from build123d import *

# Parameters (mm, degrees)
F0_W     = 381
F0_H     = 342.9
F1_DEPTH = 330.2
F2_T     = -6.35
F4_DEPTH = 12.7
F5_R     = 6.35
F6_DEPTH = 3.175
F7_R     = 12.7
F8_DEPTH = 12.7
F9_R     = 5.08


with BuildPart() as f1:
    # F0 (on Top) → F1 (new body)
    with BuildSketch(Plane.XY):
        with Locations((83.37315, 21.438057)):
            Rectangle(F0_W, F0_H)
    extrude(amount=F1_DEPTH)

    # F2
    f2_openings = [f1.faces().sort_by_distance(p)[0] for p in [
        (83.37315, 21.438057, 330.2),
    ]]
    offset(amount=F2_T, openings=f2_openings)

    # F3 (on face) → F4 (join)
    with BuildSketch(Plane.XZ.offset(150.011943)):
        Polygon((286.57315, 0), (286.57315, 342.9), (-119.82685, 342.9), (-119.82685, 0), (-107.12685, 0), (273.87315, 0), align=None)
    extrude(amount=F4_DEPTH)

    # F5 (on face) → F6 (join)
    with BuildSketch(Plane.XZ.offset(162.711943)):
        with Locations((83.37315, 171.45)):
            Circle(F5_R)
    extrude(amount=F6_DEPTH)

    # F7 (on face) → F8 (join)
    with BuildSketch(Plane.XZ.offset(165.886943)):
        with Locations((83.37315, 171.45)):
            Circle(F7_R)
    extrude(amount=F8_DEPTH)

    # F9
    f9_edges = [f1.edges().sort_by_distance(p)[0] for p in [
        (70.67315, -178.586943, 171.45),
        (70.67315, -165.886943, 171.45),
    ]]
    fillet(f9_edges, radius=F9_R)


solid = f1.part
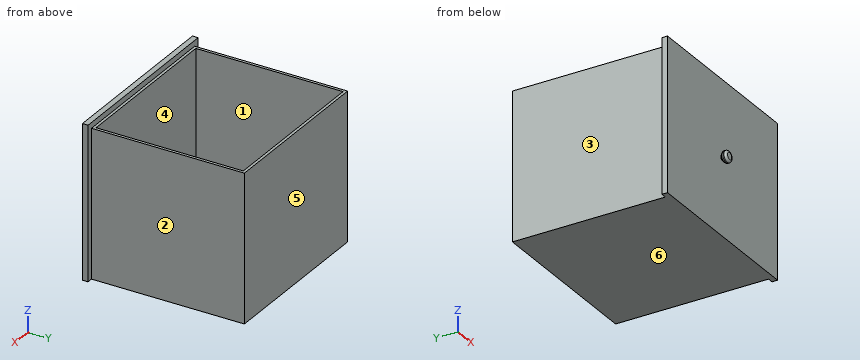
For this review, take the finished solid that the model builds, in its own axes (mm). Face numbers are marked on the shaded views. A direction names the side the tool comes from. Round coordinates to 2 decimals unless told otherwise and drop trailing zeros. Order: outer loops, then holes, each group sorted by start corner. A loop starts at its lowest first (then second) coordinate and runs counter-clockwise, first axis right, second up. Notation, with made-up numbers: (-20.5, 14) -> (38.5, 14) arc R14 cw to (38.5, 36) -> close; hole circle Ø1 at (75.5, 72). An arc over 180 degrees is marked (long way). Write item = value, one per line. Start each with the question number.
1) Take a section at A-A on z = 77. State the section outline as (x, y) points.
2) Take a section at B-B on x = 250.5. State the section outline as (y, z) points.
3) Take a section at C-C on y = 69. State the section outline as (x, z) points, plus the area to 3 significant figures.
4) Tool access review of the marked faces 1, 2 and 3: name each direction out of +Z, -Z, +X, -X, +Y, -Y from which nothing blocks a thin tool from reaching the whole face with its end or side.
5) Insertion check: pin 1 (2 mm diameter, centred on x = 199, y = 48, fed in from +Z); pin 2 (5 mm diameter, centred on y = 18, z = 285.5, fed in from -X); pin 3 (10 mm diameter, centred on x = 113, z = 169, fed in from -Y). Each pin has a flat end and moves straight along its axis. Give the tip position at first contact, or say it passes through.
6) The part is to be moulded in two halves that separate along Y. For the marked faces 4, 5 and 6, say which applies: +Y half, -Y half, draft (parallel to the pull), parting line (faces both ways), or undercut.
7) To check wall thickness, follow line 1 (X direction, y = 18.5, z = 44); line 2 (Y direction, x = 108, z = 60); line 3 (Z direction, x = -53, y = 20.5). State the ranges of each line that lie inside material, in increasing order. Write a range as from..to.
8) Take a section at D-D on z = 171.45. State the section outline as (x, y) points, plus the area to 3 significant figures.
Verdict:
q1.outline = (-119.83, -162.71) -> (286.57, -162.71) -> (286.57, -150.01) -> (273.87, -150.01) -> (273.87, 192.89) -> (-107.13, 192.89) -> (-107.13, -150.01) -> (-119.83, -150.01) -> close; hole (-100.78, -143.66) -> (267.52, -143.66) -> (267.52, 186.54) -> (-100.78, 186.54) -> close
q2.outline = (-162.71, 0) -> (192.89, 0) -> (192.89, 330.2) -> (186.54, 330.2) -> (186.54, 6.35) -> (-143.66, 6.35) -> (-143.66, 330.2) -> (-150.01, 330.2) -> (-150.01, 342.9) -> (-162.71, 342.9) -> close
q3.outline = (-107.13, 0) -> (273.87, 0) -> (273.87, 330.2) -> (267.52, 330.2) -> (267.52, 6.35) -> (-100.78, 6.35) -> (-100.78, 330.2) -> (-107.13, 330.2) -> close
q3.area = 6,530 mm2
q4.face_1 = +Z
q4.face_2 = +Z, -Z, +X, +Y
q4.face_3 = +Z, -Z, -X, +Y
q5.pin_1 = 6.35
q5.pin_2 = -107.13
q5.pin_3 = -162.71
q6.face_4 = undercut
q6.face_5 = +Y half
q6.face_6 = draft
q7.line_1 = -107.13..-100.78, 267.52..273.87
q7.line_2 = -162.71..-143.66, 186.54..192.89
q7.line_3 = 0..6.35
q8.outline = (-119.83, -162.71) -> (77.02, -162.71) -> (77.02, -165.89) -> (75.75, -165.89) arc R5.08 ccw to (70.67, -170.97) -> (70.67, -173.51) arc R5.08 ccw to (75.75, -178.59) -> (90.99, -178.59) arc R5.08 ccw to (96.07, -173.51) -> (96.07, -170.97) arc R5.08 ccw to (90.99, -165.89) -> (89.72, -165.89) -> (89.72, -162.71) -> (286.57, -162.71) -> (286.57, -150.01) -> (273.87, -150.01) -> (273.87, 192.89) -> (-107.13, 192.89) -> (-107.13, -150.01) -> (-119.83, -150.01) -> close; hole (-100.78, -143.66) -> (267.52, -143.66) -> (267.52, 186.54) -> (-100.78, 186.54) -> close
q8.area = 14,500 mm2
